Autodesk Inventor part; units mm, degrees
ref_plane "YZ Plane" through (0, 0, 0) normal (1, 0, 0) x (0, 1, 0)
ref_plane "XZ Plane" through (0, 0, 0) normal (0, 1, 0) x (-1, 0, 0)
ref_plane "XY Plane" through (0, 0, 0) normal (0, 0, 1) x (1, 0, 0)
sketch "Sketch1" plane through (0, 0, 0) normal (0, 0, 1) x (1, 0, 0)
  line L0 (-22.3155, 0) -> (133.8928, 0)
  line L1 (0, -4.6) -> (0, 6.6)
  line L2 (0, 3) -> (106.6906, 3)
  line L3 (106.6906, 3) -> (106.6906, 5)
  line L4 (106.6906, 5) -> (108.6906, 5)
  line L5 (108.6906, 5) -> (111.5774, 0)
  line L6 (0, 3) -> (3, 0)
  line L7 (0, 3) -> (0, 0)
  line L8 (111, 1) -> (111, 0)
  line L9 (0, -3) -> (3, 0)
  circle A0 centre (79.02, 0) radius 1.5
  line L10 (2.5, 3) -> (1.25, 1.75)
  line L11 (0, -3) -> (106.6906, -3)
  line L12 (2.5, -3) -> (1.25, -1.75)
  dimension "d0" = 6
  dimension "d1" = 3
  dimension "d2" = 60
  dimension "d3" = 2
  dimension "d4" = 10
  dimension "d5" = 2
  dimension "d6" = 111
  dimension "d10" = 3
  dimension "d14" = 2.5
  dimension "d16" = 31.98
revolve "Revolution1" add sketch "Sketch1" angle 360 about axis through (-10, 0, 0) along (1, 0, 0) picked at (79.1973, 0.4675) contours L6 L10 L2 L3 L4 L5 L8 L0 A0 | L2 L10 L6 | A0 L0
extrude "Extrusion1" cut sketch "Sketch1" along normal through all both and the other way through all contours L1 L6 L0 | L0 L9 L1 | L9 L12 L11 | L2 L10 L6 | A0 L0 | L0 A0
equation "\"d1\" = 0.5 * d0"
properties part number "TW1-002"
Geometry: final body of the model. Coordinates: model frame, mm. A direction names the side the tool comes from. Coordinates: 2 decimals unless noted, no trailing zeros. Loops run counter-clockwise (first coordinate to the right, second up) from the corner with the lowest first, then second, coordinate; pieces in that order, holes last. Notation, with made-up numbers: M 50.5,26.25 L 105.5,26.25 A20 cw 105.5,30.25 Z; hole C 74.5,-2.5 d6. An arc over 180 degrees is marked long. One line per item, written item: value. Start each with the question number.
1) Reachability of faces 4 (the flat face through (2, 1, 0)), 5 (the cylindrical face through (54.71, 2.77, -1.15)), 6 (the cylindrical face through (107.7, -1.08, -4.88)) from +Z, -Z, +X, -X, +Y, -Y: full face, straight path, thin tool, end or side. Return the list, or none.
2) Cut plane B-B (x = 79.02). Return loops of the section in (y, z).
3) Material intervals for L1, parallel to X at y = 0, z = -0.5; L2, parallel to Y at x = 79.02, z = -1.75; L3, parallel to X at y = -1, z = 0.75, sorted ascending. Write a range as from..to.
4) Cut plane A-A (z = 0). Return loops of the section in (x, y), then the cut area to 3 significant figures.
5) Cut plane C-C (x = 21). Return loops of the section in (y, z).
6) Pin query (flat end, axial travel): P1, Ø3, axis at y = -3.5, z = -2, coming from the +X side; P2, Ø2, axis at y = 3.5, z = 3.5, coming from the -X side; P3, Ø1.5, axis at x = 29.5, z = 1.5, coming from the -Y side. Return the tip coordinate at first contact, or that it passes through.
7) Draft query along Y for faces 1 (the conical face through (110.856, -1.249, -0.055)), 2 (the flat face through (111, 0, 0)), 3 (the flat face through (2, -1, 0)). Return one class per face: released by +Y, released by -Y, zero draft, split by the parting line, or undercut.
Evaluation:
1. face 4: +Z, -Z, -X
1. face 5: -X
1. face 6: +X, -X
2. outline: M -1.5,-2.6 L -1.5,2.6 A3 ccw Z; M 1.5,-2.6 A3 ccw 1.5,2.6 Z
3. L1: 3..77.52, 80.52..111
3. L2: -2.44..-1.5, 1.5..2.44
3. L3: 2..77.9, 80.14..110.86
4. outline: M 1.25,-1.75 L 2.5,-3 L 106.69,-3 L 106.69,-5 L 108.69,-5 L 111,-1 L 111,1 L 108.69,5 L 106.69,5 L 106.69,3 L 2.5,3 L 1.25,1.75 L 3,0 Z; hole C 79.02,0 d3
4. area: 655 mm^2
5. outline: C 0,0 d6
6. P1: x = 110.12
6. P2: x = 106.69
6. P3: y = -2.9
7. face 1: split by the parting line
7. face 2: zero draft
7. face 3: undercut
